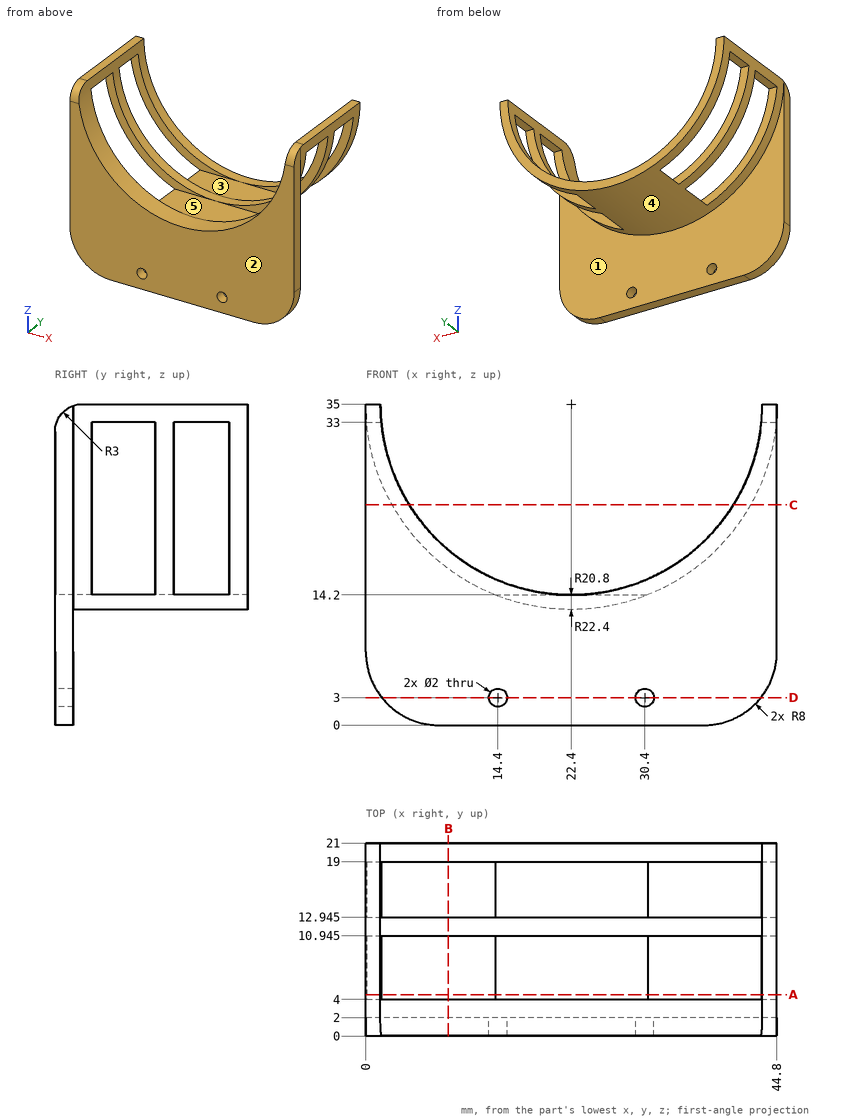
Verification items for this drawing (mm, ordinates from the low corner). A direction names the side the tool comes from. Coordinates: 2 decimals unless noted, no trailing zeros. Write each loop counter-clockwise with the first axis right and the second up, starting at its lowest first coordinate (ties: lowest second). Pieces come first, ordered by that corner, then holes. Notation, with made-up numbers: (57.5, 66) - (87.5, 66) arc R9 ccw to (87.5, 79) - close; hole circle Ø2 at (21.25, -18). An arc over 180 degrees is marked (long way). One line per question, with ' | ' between items.
Item 1: Sectioned sample at A-A on y = 4.5. Record the boundary of the cut face in (x, z).
Determined:
outline: (0, 35) arc R22.4 ccw to (0.09, 33) - (1.7, 33) arc R20.8 cw to (1.6, 35) - close; (14.09, 14.2) arc R22.4 ccw to (30.71, 14.2) - close; (43.1, 33) - (44.71, 33) arc R22.4 ccw to (44.8, 35) - (43.2, 35) arc R20.8 cw to start
Item 2: Sectioned sample at C-C on z = 24. Record the boundary of the cut face in (x, y) (1 decimal).
Determined:
outline: (0, 0) - (4.7, 0) - (4.7, 4) - (2.9, 4) - (2.9, 2) - (0, 2) - close; (2.9, 10.9) - (4.7, 10.9) - (4.7, 12.9) - (2.9, 12.9) - close; (2.9, 19) - (4.7, 19) - (4.7, 21) - (2.9, 21) - close; (40.1, 0) - (44.8, 0) - (44.8, 2) - (41.9, 2) - (41.9, 4) - (40.1, 4) - close; (40.1, 10.9) - (41.9, 10.9) - (41.9, 12.9) - (40.1, 12.9) - close; (40.1, 19) - (41.9, 19) - (41.9, 21) - (40.1, 21) - close
Item 3: Mould release check, pull along Y, two halves, no side actions. Record for the marked faces 1, 2 and 3: pulls with the +Y half, pulls with the -Y half, needs draft (parallel to the pull), parting line crosses it, or undercut.
Determined:
face 1: pulls with the +Y half | face 2: pulls with the -Y half | face 3: undercut
Item 4: Access from +Z, -Z, +X, -X, +Y, -Y to the whole of each face (thin tool, end or side, straight path). Record for the marked faces 4 and 5.
Determined:
face 4: -Z, +Y | face 5: +Z, +X, -X
Item 5: Sectioned sample at B-B on x = 9. Give the number of separate pieces and of enclosed holes in the cut face.
Determined:
separate pieces: 3 | enclosed holes: 0
Item 6: Thickness scan on line 1 (X direction, y = 0.65, z = 3) (1 decimal); line 2 (X direction, y = 1.5, z = 34.5); line 3 (Z direction, x = 22, y = 9.5). Record the ranges inside material, lowest first. Write a range as [from, to].
Determined:
line 1: x = [1.8, 13.4], [15.4, 29.4], [31.4, 43] | line 2: x = [0, 1.61], [43.19, 44.8] | line 3: z = [12.6, 14.2]
Item 7: Gauge pin test, flat ends, axial feed: P1, Ø2.5, axis at x = 14.4, z = 3, coming from the +Y side; P2, Ø3.5, axis at x = 20.5, y = 9, coming from the +Z side; P3, Ø1.8, axis at x = 1, y = 8.5, coming from the -Z side. Record the tip position at first contact, or that the pin passes through.
Determined:
P1: stops at y = 2 | P2: stops at z = 14.2 | P3: stops at z = 33
Item 8: Sectioned sample at D-D on z = 3. Record the boundary of the cut face in (x, y) (3 decimals).
Determined:
outline: (1.755, 0) - (13.4, 0) - (13.4, 2) - (1.755, 2) - close; (15.4, 0) - (29.4, 0) - (29.4, 2) - (15.4, 2) - close; (31.4, 0) - (43.045, 0) - (43.045, 2) - (31.4, 2) - close
